```python
from build123d import *

# Parameters (mm, degrees)
BOSS_EXTRUDE1_DEPTH = 3
SKETCH3_W           = 3
SKETCH3_H           = 22.5
BOSS_EXTRUDE2_DEPTH = 25
SKETCH4_R           = 4
CUT_EXTRUDE1_DEPTH  = 3


with BuildPart() as part:
    # Sketch2 → Boss-Extrude1 (new body)
    with BuildSketch(Plane(origin=(0, 0, 0), x_dir=(1, 0, 0), z_dir=(0, 1, 0))):
        with BuildLine():
            Line((-15.860247962, 17.20906431), (-13.694996915, 20.301363277))
            ThreePointArc((-13.694996915, 20.301363277), (-19.875283017, 22.25), (-26.055569119, 20.301363277))
            Line((-26.055569119, 20.301363277), (-26.055569119, 34.118363277))
            Line((-26.055569119, 34.118363277), (-26.055569119, 59.118363277))
            Line((-26.055569119, 59.118363277), (-16.055569119, 59.118363277))
            Line((-16.055569119, 59.118363277), (-16.055569119, 34.118363277))
            Line((-16.055569119, 34.118363277), (26.055569119, 34.118363277))
            Line((26.055569119, 34.118363277), (26.055569119, 20.301363277))
            ThreePointArc((26.055569119, 20.301363277), (19.875283017, 22.25), (13.694996915, 20.301363277))
            Line((13.694996915, 20.301363277), (15.860247962, 17.20906431))
            ThreePointArc((15.860247962, 17.20906431), (13.666207185, 14.707240293), (12.875283017, 11.475))
            ThreePointArc((12.875283017, 11.475), (10.090653959, 8.727908609), (6.180286102, 8.826363277))
            ThreePointArc((6.180286102, 8.826363277), (0, 10.775), (-6.180286102, 8.826363277))
            ThreePointArc((-6.180286102, 8.826363277), (-10.090653959, 8.727908609), (-12.875283017, 11.475))
            ThreePointArc((-12.875283017, 11.475), (-13.666207185, 14.707240293), (-15.860247962, 17.20906431))
        make_face()
    extrude(amount=BOSS_EXTRUDE1_DEPTH)

    # Sketch3 → Boss-Extrude2 (add)
    with BuildSketch(Plane.XZ):
        with Locations((-24.555569119, -47.868363277)):
            Rectangle(SKETCH3_W, SKETCH3_H)
    extrude(amount=BOSS_EXTRUDE2_DEPTH)

    # Sketch4 → Cut-Extrude1 (cut)
    with BuildSketch(Plane.ZY.offset(26.055569119)):
        with Locations((-47.868363277, -15)):
            Circle(SKETCH4_R)
    extrude(amount=-CUT_EXTRUDE1_DEPTH, mode=Mode.SUBTRACT)


solid = part.part
```
Here's how the part is built. I have some questions about the finished solid (model axes, mm). A direction names the side the tool comes from. Coordinates: 2 decimals unless noted, no trailing zeros. Write each loop counter-clockwise with the first axis right and the second up, starting at its lowest first coordinate (ties: lowest second). Pieces come first, ordered by that corner, then holes. Notation, with made-up numbers: (82, 69.5) - (138, 69.5) arc R15 ccw to (138, 97.5) - close; hole circle Ø4 at (-4.75, 27.25). An arc over 180 degrees is marked (long way). One line per item, written item: value.
1) I need wall thicknesses on line 1 along X through (y, z) = (1.5, -51); line 2 along Y through (x, z) = (1.5, -32); line 3 along X through (y, z) = (-13.5, -44). Which ranges of each line are inside material? Lowest first, please.
Model answer:
line 1: x = -26.06 to -16.06
line 2: y = 0 to 3
line 3: x = -26.06 to -23.06
2) I'm going to push flat-ended pins straight in: P1, Ø15, axis at x = -11, z = -28.5, coming from the -Y side; P2, Ø3.5, axis at x = 2, y = 2, coming from the -Z side; P3, Ø10, axis at x = -18, z = -15, coming from the +Y side; P4, Ø2.5, axis at y = 1.5, z = -46.5, coming from the +X side. Where does each tip first touch, or does it pass through?
Model answer:
P1: stops at y = 0
P2: stops at z = -34.12
P3: stops at y = 3
P4: stops at x = -16.06
3) Suppose I cut it at C-C on z = -24. Write out the boundary of the cut face in (x, y).
Model answer:
outline: (-26.06, 0) - (26.06, 0) - (26.06, 3) - (-26.06, 3) - close
4) Suppose I cut it at A-A on y = -15. Write out the boundary of the cut face in (x, z).
Model answer:
outline: (-26.06, -59.12) - (-23.06, -59.12) - (-23.06, -51.87) - (-26.06, -51.87) - close; (-26.06, -43.87) - (-23.06, -43.87) - (-23.06, -36.62) - (-26.06, -36.62) - close
5) We'd pull the mould along X, two halves only. Please class faces 1 (the cylindrical face through (10.143, 1.479, -8.749)), 2 (the flat face through (14.76, 1.48, -18.78)), 3 (the flat face through (-26.056, -11, -49)), 4 (the cylindrical face through (0.092, 1.479, -10.775)): pulls with the +X half, pulls with the -X half, needs draft (parallel to the pull), parting line crosses it, or undercut.
Model answer:
face 1: undercut
face 2: pulls with the +X half
face 3: pulls with the -X half
face 4: undercut
6) On a 3-axis mill with a long thin cutter (end or side, diameter ignored), from which of +Z, -Z, +X, -X, +Y, -Y can I reach the whole of each face in a straight line? I mean faces 5 (the flat face through (-25, -12, -36.618)), 6 (the flat face through (-14.793, 1.479, -18.734)), 7 (the cylindrical face through (19.97, 1.48, -22.25)), 8 (the flat face through (-16.056, 1, -47)), 9 (the flat face through (-23.056, -10, -48)). Say none if no direction works.
Model answer:
face 5: +Z, +X, -X, -Y
face 6: -X, +Y, -Y
face 7: +Y, -Y
face 8: -Z, +X, +Y, -Y
face 9: +Z, -Z, +X, -Y
7) Suppose I cut it at B-B on y = -8.75. Write out the boundary of the cut face in (x, z).
Model answer:
outline: (-26.06, -59.12) - (-23.06, -59.12) - (-23.06, -36.62) - (-26.06, -36.62) - close
